```python
from build123d import *

# Parameters (mm, degrees)
SKETCH1_R           = 25
BOSS_EXTRUDE1_DEPTH = 5


with BuildPart() as part:
    # Sketch1 → Boss-Extrude1 (new, symmetric)
    with BuildSketch(Plane(origin=(0, 0, 0), x_dir=(1, 0, 0), z_dir=(0, 1, 0))):
        with BuildLine():
            Line((10.182093062, 37.647376813), (12.49472571, 43.230565916))
            ThreePointArc((12.49472571, 43.230565916), (17.220754456, 41.574578963), (21.733521035, 39.403731592))
            Line((21.733521035, 39.403731592), (19.420888387, 33.820542489))
            ThreePointArc((19.420888387, 33.820542489), (21.667239088, 32.42731488), (23.814054756, 30.885122568))
            Line((23.814054756, 30.885122568), (28.087242696, 35.158310508))
            ThreePointArc((28.087242696, 35.158310508), (31.819805153, 31.819805153), (35.158310508, 28.087242696))
            Line((35.158310508, 28.087242696), (30.885122568, 23.814054756))
            ThreePointArc((30.885122568, 23.814054756), (32.42731488, 21.667239088), (33.820542489, 19.420888387))
            Line((33.820542489, 19.420888387), (39.403731592, 21.733521035))
            ThreePointArc((39.403731592, 21.733521035), (41.574578963, 17.220754456), (43.230565916, 12.49472571))
            Line((43.230565916, 12.49472571), (37.647376813, 10.182093062))
            ThreePointArc((37.647376813, 10.182093062), (38.250625936, 7.608522559), (38.678159212, 5))
            Line((38.678159212, 5), (44.72135955, 5))
            ThreePointArc((44.72135955, 5), (45, 0), (44.72135955, -5))
            Line((44.72135955, -5), (38.678159212, -5))
            ThreePointArc((38.678159212, -5), (38.250625936, -7.608522559), (37.647376813, -10.182093062))
            Line((37.647376813, -10.182093062), (43.230565916, -12.49472571))
            ThreePointArc((43.230565916, -12.49472571), (41.574578963, -17.220754456), (39.403731592, -21.733521035))
            Line((39.403731592, -21.733521035), (33.820542489, -19.420888387))
            ThreePointArc((33.820542489, -19.420888387), (32.42731488, -21.667239088), (30.885122568, -23.814054756))
            Line((30.885122568, -23.814054756), (35.158310508, -28.087242696))
            ThreePointArc((35.158310508, -28.087242696), (31.819805153, -31.819805153), (28.087242696, -35.158310508))
            Line((28.087242696, -35.158310508), (23.814054756, -30.885122568))
            ThreePointArc((23.814054756, -30.885122568), (21.667239088, -32.42731488), (19.420888387, -33.820542489))
            Line((19.420888387, -33.820542489), (21.733521035, -39.403731592))
            ThreePointArc((21.733521035, -39.403731592), (17.220754456, -41.574578963), (12.49472571, -43.230565916))
            Line((12.49472571, -43.230565916), (10.182093062, -37.647376813))
            ThreePointArc((10.182093062, -37.647376813), (7.608522559, -38.250625936), (5, -38.678159212))
            Line((5, -38.678159212), (5, -44.72135955))
            ThreePointArc((5, -44.72135955), (0, -45), (-5, -44.72135955))
            Line((-5, -44.72135955), (-5, -38.678159212))
            ThreePointArc((-5, -38.678159212), (-7.608522559, -38.250625936), (-10.182093062, -37.647376813))
            Line((-10.182093062, -37.647376813), (-12.49472571, -43.230565916))
            ThreePointArc((-12.49472571, -43.230565916), (-17.220754456, -41.574578963), (-21.733521035, -39.403731592))
            Line((-21.733521035, -39.403731592), (-19.420888387, -33.820542489))
            ThreePointArc((-19.420888387, -33.820542489), (-21.667239088, -32.42731488), (-23.814054756, -30.885122568))
            Line((-23.814054756, -30.885122568), (-28.087242696, -35.158310508))
            ThreePointArc((-28.087242696, -35.158310508), (-31.819805153, -31.819805153), (-35.158310508, -28.087242696))
            Line((-35.158310508, -28.087242696), (-30.885122568, -23.814054756))
            ThreePointArc((-30.885122568, -23.814054756), (-32.42731488, -21.667239088), (-33.820542489, -19.420888387))
            Line((-33.820542489, -19.420888387), (-39.403731592, -21.733521035))
            ThreePointArc((-39.403731592, -21.733521035), (-41.574578963, -17.220754456), (-43.230565916, -12.49472571))
            Line((-43.230565916, -12.49472571), (-37.647376813, -10.182093062))
            ThreePointArc((-37.647376813, -10.182093062), (-38.250625936, -7.608522559), (-38.678159212, -5))
            Line((-38.678159212, -5), (-44.72135955, -5))
            ThreePointArc((-44.72135955, -5), (-45, 0), (-44.72135955, 5))
            Line((-44.72135955, 5), (-38.678159212, 5))
            ThreePointArc((-38.678159212, 5), (-38.250625936, 7.608522559), (-37.647376813, 10.182093062))
            Line((-37.647376813, 10.182093062), (-43.230565916, 12.49472571))
            ThreePointArc((-43.230565916, 12.49472571), (-41.574578963, 17.220754456), (-39.403731592, 21.733521035))
            Line((-39.403731592, 21.733521035), (-33.820542489, 19.420888387))
            ThreePointArc((-33.820542489, 19.420888387), (-32.42731488, 21.667239088), (-30.885122568, 23.814054756))
            Line((-30.885122568, 23.814054756), (-35.158310508, 28.087242696))
            ThreePointArc((-35.158310508, 28.087242696), (-31.819805153, 31.819805153), (-28.087242696, 35.158310508))
            Line((-28.087242696, 35.158310508), (-23.814054756, 30.885122568))
            ThreePointArc((-23.814054756, 30.885122568), (-21.667239088, 32.42731488), (-19.420888387, 33.820542489))
            Line((-19.420888387, 33.820542489), (-21.733521035, 39.403731592))
            ThreePointArc((-21.733521035, 39.403731592), (-17.220754456, 41.574578963), (-12.49472571, 43.230565916))
            Line((-12.49472571, 43.230565916), (-10.182093062, 37.647376813))
            ThreePointArc((-10.182093062, 37.647376813), (-7.608522559, 38.250625936), (-5, 38.678159212))
            Line((-5, 38.678159212), (-5, 44.72135955))
            ThreePointArc((-5, 44.72135955), (0, 45), (5, 44.72135955))
            Line((5, 44.72135955), (5, 38.678159212))
            ThreePointArc((5, 38.678159212), (7.608522559, 38.250625936), (10.182093062, 37.647376813))
        make_face()
        with Locations(Location((0, 0, 0), (0, 0, 270))):
            Circle(SKETCH1_R, mode=Mode.SUBTRACT)
    extrude(amount=BOSS_EXTRUDE1_DEPTH, both=True)


solid = part.part
```
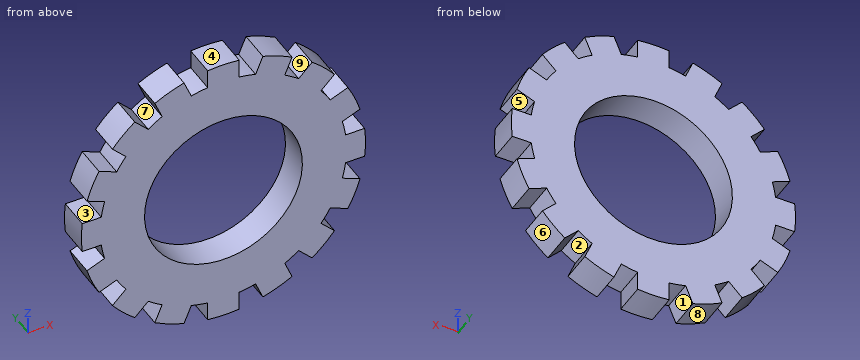
Input: part model. Units: mm. Frame: model coordinates. Face numbers are marked on the shaded views. A direction names the side the tool comes from. Round coordinates to 2 decimals unless told otherwise and drop trailing zeros. Loops run counter-clockwise (first coordinate to the right, second up) from the corner with the lowest first, then second, coordinate; pieces in that order, holes last. Notation, with made-up numbers: (11, 47) -> (32, 47) arc R15 cw to (32, 54) -> close; hole circle Ø9 at (-1, 68.25). An arc over 180 degrees is marked (long way). Write each question's results on one line, items separated by ' | '.
1. Set-up query: the marked faces 1, 2, 3, 4 and 5. Return all of +Z, -Z, +X, -X, +Y, -Y with unobstructed straight access to the full face (end or side cutting, diameter ignored); none if empty.
Geometry results:
face 1: -Z, +Y, -Y | face 2: +Y, -Y | face 3: -X, +Y, -Y | face 4: +Z, +Y, -Y | face 5: +X, +Y, -Y
2. Ray query, line 1 (X direction, y = 1.5, z = 33); line 2 (Z direction, x = -34.5, y = 4); line 3 (X direction, y = 1, z = -32). Return the intervals inside material, ascending. Write a range as from..to.
Geometry results:
line 1: -30.59..-25.93, -20.78..20.78, 25.93..30.59 | line 2: -28.89..-27.43, -19.7..19.7, 27.43..28.89 | line 3: -31.64..-24.93, -22.29..22.29, 24.93..31.64
3. Section A-A (z = 0). Return loops of the section in (x, y).
Geometry results:
outline: (-45, -5) -> (-25, -5) -> (-25, 5) -> (-45, 5) -> close; (25, -5) -> (45, -5) -> (45, 5) -> (25, 5) -> close
4. First-contact query: P1, Ø5, axis at y = 3, z = -13, coming from the -X side; P2, Ø3, axis at x = -42, y = 2.5, coming from the +Z side; P3, Ø5, axis at y = -2.5, z = 31, coming from the -X side. Flat tips, straight axial feed; report the tip coordinate or a pass-through.
Geometry results:
P1: x = -43.23 | P2: z = 19.62 | P3: x = -34.82
5. Section B-B (x = 0). Return loops of the section in (y, z), and give its area (3 significant figures).
Geometry results:
outline: (-5, -45) -> (5, -45) -> (5, -25) -> (-5, -25) -> close; (-5, 25) -> (5, 25) -> (5, 45) -> (-5, 45) -> close | area: 400 mm2
6. Mould query, pull axis X, two halves, no side actions, for the marked faces 6, 7, 8 and 9. Classes: +X half, -X half, draft (parallel to the pull), parting line (faces both ways), or undercut.
Geometry results:
face 6: +X half | face 7: undercut | face 8: -X half | face 9: undercut
